Part model, mm, in its own coordinate system. A direction names the side the tool comes from. Coordinates: 2 decimals unless noted, no trailing zeros. Write each loop counter-clockwise with the first axis right and the second up, starting at its lowest first coordinate (ties: lowest second). Pieces come first, ordered by that corner, then holes. Notation, with made-up numbers: (36.5, 67) -> (53.5, 67) arc R19 ccw to (53.5, 99) -> close; hole circle Ø10 at (-10.5, -16). An arc over 180 degrees is marked (long way). Write item = value, one per line.
from build123d import *

# Parameters (mm, degrees)
SKETCH1_R           = 7.5
BOSS_EXTRUDE1_DEPTH = 5.08
SKETCH2_W           = 5.08
SKETCH2_H           = 10
SKETCH2_H_2         = 15
CUT_EXTRUDE1_DEPTH  = 5.08


with BuildPart() as part:
    # Sketch1 → Boss-Extrude1 (new body)
    with BuildSketch(Plane(origin=(0, 0, 0), x_dir=(1, 0, 0), z_dir=(0, 1, 0))):
        Polygon((12, -32.5), (-12, -32.5), (-12, 32.5), (-12, 62.5), (12, 62.5), (12, 32.5), align=None)
        with Locations((0, 32.5)):
            Circle(SKETCH1_R, mode=Mode.SUBTRACT)
    extrude(amount=BOSS_EXTRUDE1_DEPTH)

    # Sketch2 → Cut-Extrude1 (cut)
    with BuildSketch(Plane(origin=(0, 5.08, 0), x_dir=(1, 0, 0), z_dir=(0, 1, 0))):
        with Locations((-9.46, 42.5)):
            Rectangle(SKETCH2_W, SKETCH2_H)
        with Locations((-9.46, -15)):
            Rectangle(SKETCH2_W, SKETCH2_H_2)
        with Locations((-9.46, 10)):
            Rectangle(SKETCH2_W, SKETCH2_H_2)
    cut_extrude1 = extrude(amount=-CUT_EXTRUDE1_DEPTH, mode=Mode.SUBTRACT)

    # Mirror2: Cut-Extrude1 across plane
    add(cut_extrude1.mirror(Plane(origin=(0, 0, 0), x_dir=(0, 0, 1), z_dir=(1, 0, 0))), mode=Mode.SUBTRACT)


solid = part.part
Q1. Saw through at C-C on z = -32.5. Give the cut face in (x, y).
Model answer:
outline = (-12, 0) -> (-7.5, 0) -> (-7.5, 5.08) -> (-12, 5.08) -> close; (7.5, 0) -> (12, 0) -> (12, 5.08) -> (7.5, 5.08) -> close
Q2. Pin check, flat tips, straight feed: pin 1 (3 mm diameter, centred on y = 0.5, z = -41, fed in from -X); pin 2 (1.5 mm diameter, centred on y = 3, z = -7, fed in from +X). Stop position of each tip, or through.
Model answer:
pin_1 = -6.92
pin_2 = 6.92
Q3. Saw through at B-B on x = 10. Give the cut face in (y, z).
Model answer:
outline = (0, -62.5) -> (5.08, -62.5) -> (5.08, -47.5) -> (0, -47.5) -> close; (0, -37.5) -> (5.08, -37.5) -> (5.08, -17.5) -> (0, -17.5) -> close; (0, -2.5) -> (5.08, -2.5) -> (5.08, 7.5) -> (0, 7.5) -> close; (0, 22.5) -> (5.08, 22.5) -> (5.08, 32.5) -> (0, 32.5) -> close
Q4. Which spindle directions (+Z, -Z, +X, -X, +Y, -Y) get a long thin tool onto all of the face, cutting with end or side? Do faces 5 (the face through (-6.92, 3, -42)), 6 (the face through (6.92, 3, -10)), 7 (the face through (-12, 3, 2)). Say none if no direction does.
Model answer:
face_5 = -X, +Y, -Y
face_6 = +X, +Y, -Y
face_7 = +Z, -Z, -X, +Y, -Y
Q5. Probe line 1 (Z direction, x = 11.25, y = 2.95); line 2 (X direction, y = 2.05, z = -32.5); line 3 (Z direction, x = 0, y = 3.45). List the from-to ranges inside material, lowest first. Write a range as from..to.
Model answer:
line_1 = -62.5..-47.5, -37.5..-17.5, -2.5..7.5, 22.5..32.5
line_2 = -12..-7.5, 7.5..12
line_3 = -62.5..-40, -25..32.5
Q6. Mould opens along Z. For faces 1 (the face through (9, 3, -2.5)), 2 (the face through (9, 3, 7.5)), 3 (the face through (12, 3, 3)), 4 (the face through (0, 3, -62.5)) say: released by +Z, released by -Z, zero draft, split by the parting line, or undercut.
Model answer:
face_1 = undercut
face_2 = undercut
face_3 = zero draft
face_4 = released by -Z
Q7. Saw through at A-A on x = 0. Give the cut face in (y, z).
Model answer:
outline = (0, -62.5) -> (5.08, -62.5) -> (5.08, -40) -> (0, -40) -> close; (0, -25) -> (5.08, -25) -> (5.08, 32.5) -> (0, 32.5) -> close
